Check sheet for the drawn part. Datum: minimum x, y, z corner. Units: mm. A direction names the side the tool comes from. Coordinates: 2 decimals unless noted, no trailing zeros. Loops run counter-clockwise (first coordinate to the right, second up) from the corner with the lowest first, then second, coordinate; pieces in that order, holes last. Notation, with made-up numbers: (44, -32) -> (70, -32) arc R25 ccw to (70, 5) -> close; hole circle Ø10 at (38.25, 15.5). An arc over 180 degrees is marked (long way). Use CSV: the item, a comma, the result in double quotes. Start each with the question number.
1. Gauge pin test, flat ends, axial feed: pin 1 (1 mm diameter, centred on x = 59.5, y = 14, fed in from -Z); pin 2 (1 mm diameter, centred on x = 57.5, y = 16.5, fed in from -Z); pin 3 (10.5 mm diameter, centred on x = 37, z = 6, fed in from +Y). Record the tip position at first contact, or that the pin passes through.
2. Sectioned sample at C-C, the plane y = 16.5. Record the cut outline in (x, z).
3. Thickness scan on L1, parallel to Y at x = 23, z = 5; L2, parallel to Y at x = 17, z = 11.5; L3, parallel to Z at x = 67.5, y = 12.25. Record the ranges inside material, lowest first.
4. Set-up check for the marked faces 1 and 2: record each of +Z, -Z, +X, -X, +Y, -Y from which the full face is reachable in a straight line by a thin tool's end or side.
5. Sectioned sample at A-A, the plane x = 41. Record the cut outline in (y, z).
6. Sectioned sample at B-B, the plane z = 6. Record the cut outline in (x, y).
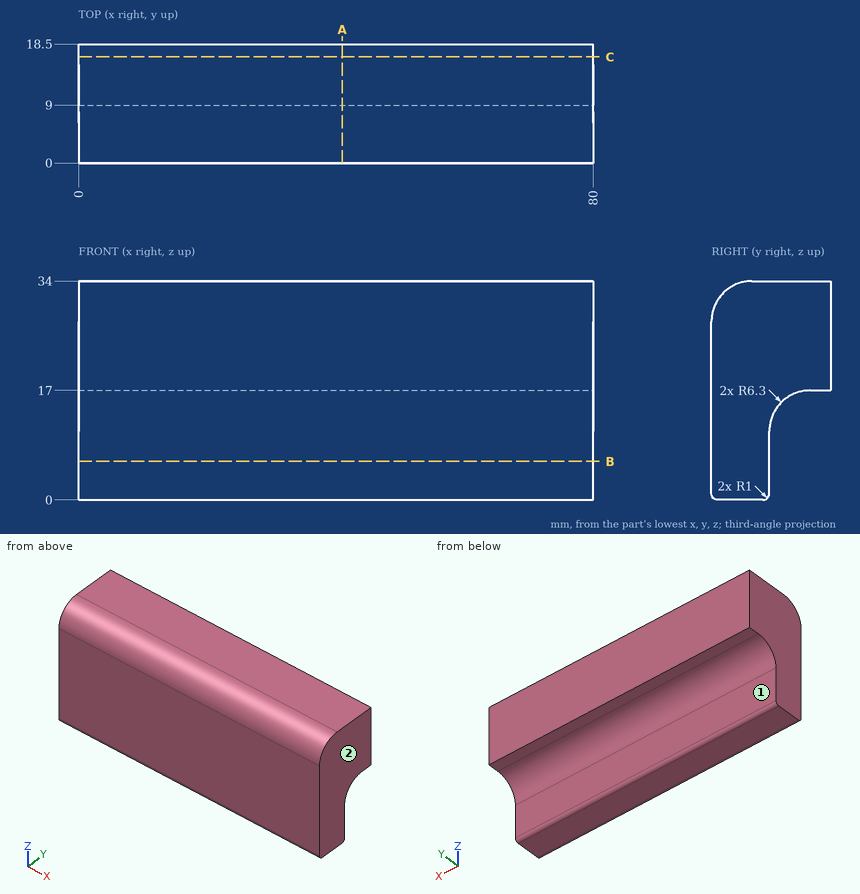
Completed:
1,pin 1,"z = 16.74"
1,pin 2,"z = 17"
1,pin 3,"y = 9.02"
2,outline,"(0, 17) -> (80, 17) -> (80, 34) -> (0, 34) -> close"
3,L1,"0 to 9"
3,L2,"0 to 9.05"
3,L3,"16.21 to 34"
4,face 1,"-Z, +X, -X, +Y"
4,face 2,"+Z, -Z, +X, +Y, -Y"
5,outline,"(0, 1) arc R1 ccw to (1, 0) -> (8, 0) arc R1 ccw to (9, 1) -> (9, 10.7) arc R6.3 cw to (15.3, 17) -> (18.5, 17) -> (18.5, 34) -> (6.3, 34) arc R6.3 ccw to (0, 27.7) -> close"
6,outline,"(0, 0) -> (80, 0) -> (80, 9) -> (0, 9) -> close"
